Geometry check sheet. Reference: the model listing, model coordinates, mm. Face numbers are marked on the shaded views. A direction names the side the tool comes from. Round coordinates to 2 decimals unless told otherwise and drop trailing zeros. Order: outer loops, then holes, each group sorted by start corner. A loop starts at its lowest first (then second) coordinate and runs counter-clockwise, first axis right, second up.
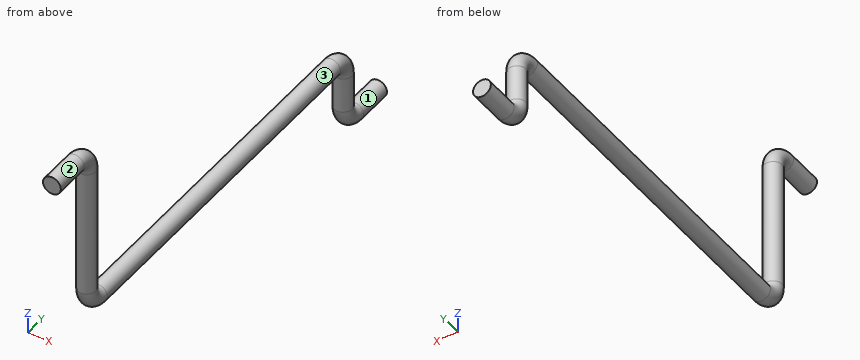
```python
from build123d import *

# Parameters (mm, degrees)
SKETCH2_R = 0.5


with BuildPart() as part:
    # Sweep1: sweep along a path in Sketch1
    with BuildLine(Plane(origin=(0, 0, 0), x_dir=(0, 0, -1), z_dir=(1, 0, 0))) as sweep1_path:
        Line((0, 0), (0, 2))
        ThreePointArc((0, 2), (0.292893219, 2.707106781), (1, 3))
        Line((1, 3), (8.22, 3))
        ThreePointArc((8.22, 3), (8.927106781, 3.292893219), (9.22, 4))
        Line((9.22, 4), (9.22, 24))
        ThreePointArc((9.22, 24), (9.512893219, 24.707106781), (10.22, 25))
        Line((10.22, 25), (12.22, 25))
        ThreePointArc((12.22, 25), (12.927106781, 25.292893219), (13.22, 26))
        Line((13.22, 26), (13.22, 28))
    # Sketch2 → Sweep1 (sweep)
    with BuildSketch(Plane(origin=(0, 0, 0), x_dir=(1, 0, 0), z_dir=(0, 1, 0))):
        Circle(SKETCH2_R)
    sweep(path=sweep1_path.line)


solid = part.part
```
(1) Sectioned sample at A-A, the plane x = 0.3. Record the cut outline in (y, z).
Returned:
outline: (0, -0.4) - (2, -0.4) arc R0.6 cw to (2.6, -1) - (2.6, -8.22) arc R1.4 ccw to (4, -9.62) - (24, -9.62) arc R0.6 cw to (24.6, -10.22) - (24.6, -12.22) arc R1.4 ccw to (26, -13.62) - (28, -13.62) - (28, -12.82) - (26, -12.82) arc R0.6 cw to (25.4, -12.22) - (25.4, -10.22) arc R1.4 ccw to (24, -8.82) - (4, -8.82) arc R0.6 cw to (3.4, -8.22) - (3.4, -1) arc R1.4 ccw to (2, 0.4) - (0, 0.4) - close
(2) Material ranges on line 1 (Y direction, x = -0.05, z = -11); line 2 (X direction, y = 3.75, z = -9.25); line 3 (Y direction, x = 0.05, z = -5.5), recorded low to high.
Returned:
line 1: y = 24.5 to 25.5
line 2: x = -0.5 to 0.5
line 3: y = 2.5 to 3.5
(3) Set-up check for the marked faces 1, 2 and 3: record each of +Z, -Z, +X, -X, +Y, -Y from which the full face is reachable in a straight line by a thin tool's end or side.
Returned:
face 1: +Y
face 2: -Y
face 3: none
(4) Sectioned sample at B-B, the plane z = -6. Record the cut outline in (x, y), and give its area (3 significant figures).
Returned:
outline: circle Ø1 at (0, 3)
area: 0.785 mm2
(5) Sectioned sample at C-C, the plane y = 15.5. Record the cut outline in (x, z), and give its area (3 significant figures).
Returned:
outline: circle Ø1 at (0, -9.22)
area: 0.785 mm2
